from build123d import *

# Parameters (mm, degrees)
SKETCH1_W               = 154.5
SKETCH1_H               = 30
SKETCH1_W_2             = 34.5
SKETCH1_H_2             = 20
BOSS_EXTRUDE2_DEPTH     = 1
BOSS_EXTRUDE5_DEPTH     = 24
SKETCH5_W               = 3.2
SKETCH5_H               = 10
SKETCH5_H_2             = 8
SKETCH5_H_3             = 6
SKETCH5_H_4             = 4
SKETCH5_W_2             = 3
BOSS_EXTRUDE6_DEPTH     = 24
SKETCH6_W               = 28.5
SKETCH6_H               = 20
BOSS_EXTRUDE7_DEPTH     = 15
BOSS_EXTRUDE8_DEPTH     = 10
SKETCH9_W               = 8
SKETCH9_H               = 3
BOSS_EXTRUDE9_DEPTH     = 25
SKETCH10_R              = 2
CUT_EXTRUDE1_DEPTH      = 8
SKETCH11_W              = 32
SKETCH11_H              = 24
SKETCH11_W_2            = 34.7
CUT_EXTRUDE2_DEPTH      = 8
FILLET1_R               = 10
SKETCH13_W              = 15
SKETCH13_H              = 6
BOSS_EXTRUDE10_DEPTH    = 25
SKETCH15_W              = 6.4
SKETCH15_H              = 5
CUT_EXTRUDE3_DEPTH      = 7
CUT_EXTRUDE4_DEPTH      = 170.470498908
CUT_EXTRUDE4_DEPTH_BACK = 170.470498908
CHAMFER1_SIZE           = 6
SKETCH17_W              = 34.5
SKETCH17_H              = 3
BOSS_EXTRUDE11_DEPTH    = 10
CHAMFER2_SIZE           = 10


# Some blends are built 0.0001 mm under size
with BuildPart() as part:
    # Sketch1 → Boss-Extrude2 (new body)
    with BuildSketch(Plane(origin=(0, 0, 0), x_dir=(1, 0, 0), z_dir=(0, 1, 0))):
        with Locations((77.25, 15)):
            Rectangle(SKETCH1_W, SKETCH1_H)
        with Locations((137.25, -10)):
            Rectangle(SKETCH1_W_2, SKETCH1_H_2)
    extrude(amount=BOSS_EXTRUDE2_DEPTH)

    # Sketch2 → Boss-Extrude5 (add)
    with BuildSketch(Plane(origin=(0, 1, 0), x_dir=(1, 0, 0), z_dir=(0, 1, 0))):
        Polygon((3, 27), (0, 27), (0, 30), (154.5, 30), (154.5, 27), (151.5, 27), align=None)
        Polygon((0, 0), (120, 0), (120, -20), (154.5, -20), (154.5, 3), (151.5, 3), (151.5, -17), (123, -17), (123, 3), (3, 3), (0, 3), align=None)
    extrude(amount=BOSS_EXTRUDE5_DEPTH)

    # Sketch5 → Boss-Extrude6 (add)
    with BuildSketch(Plane.XY.offset(-27)):
        with Locations((9.6, 6)):
            Rectangle(SKETCH5_W, SKETCH5_H)
        with Locations((44.8, 5)):
            Rectangle(SKETCH5_W, SKETCH5_H_2)
        with Locations((80, 4)):
            Rectangle(SKETCH5_W, SKETCH5_H_3)
        with Locations((115.2, 3)):
            Rectangle(SKETCH5_W, SKETCH5_H_4)
        with Locations((153, 3)):
            Rectangle(SKETCH5_W_2, SKETCH5_H_4)
    extrude(amount=BOSS_EXTRUDE6_DEPTH)

    # Sketch6 → Boss-Extrude7 (add)
    with BuildSketch(Plane(origin=(0, 1, 0), x_dir=(1, 0, 0), z_dir=(0, 1, 0))):
        with Locations((137.25, -7)):
            Rectangle(SKETCH6_W, SKETCH6_H)
    extrude(amount=BOSS_EXTRUDE7_DEPTH)

    # Sketch7 → Boss-Extrude8 (add)
    with BuildSketch(Plane(origin=(0, 25, 0), x_dir=(1, 0, 0), z_dir=(0, 1, 0))):
        Polygon((110, 3), (110, 0), (122, 0), (122, -20), (152.5, -20), (152.5, 0), (162.5, 0), (162.5, 3), (151.5, 3), (151.5, -17), (123, -17), (123, 3), align=None)
    extrude(amount=BOSS_EXTRUDE8_DEPTH)

    # Sketch9 → Boss-Extrude9 (add)
    with BuildSketch(Plane.XZ.offset(-25)):
        with Locations((158.5, -1.5)):
            Rectangle(SKETCH9_W, SKETCH9_H)
    extrude(amount=BOSS_EXTRUDE9_DEPTH)

    # Sketch10 → Cut-Extrude1 (cut)
    with BuildSketch(Plane(origin=(0, 0, -3), x_dir=(-1, 0, 0), z_dir=(0, 0, -1))):
        with Locations((-120, 30)):
            Circle(SKETCH10_R)
        with Locations((-154.5, 30)):
            Circle(SKETCH10_R)
    extrude(amount=-CUT_EXTRUDE1_DEPTH, mode=Mode.SUBTRACT)

    # Sketch11 → Cut-Extrude2 (cut)
    with BuildSketch(Plane(origin=(0, 1, 0), x_dir=(1, 0, 0), z_dir=(0, 1, 0))):
        with Locations((27.2, 15)):
            Rectangle(SKETCH11_W, SKETCH11_H)
        with Locations((62.4, 15)):
            Rectangle(SKETCH11_W, SKETCH11_H)
        with Locations((97.6, 15)):
            Rectangle(SKETCH11_W, SKETCH11_H)
        with Locations((134.15, 15)):
            Rectangle(SKETCH11_W_2, SKETCH11_H)
    extrude(amount=-CUT_EXTRUDE2_DEPTH, mode=Mode.SUBTRACT)

    # Fillet1
    # the kernel refuses this fillet: 10 mm, written as the material it adds along each edge
    with BuildSketch(Plane(origin=(46.4, 0, -3), x_dir=(1, 0, 0), z_dir=(0, 1, 0)), Plane(origin=(43.2, 9, -3), x_dir=(-1, 0, 0), z_dir=(0, -1, 0)), Plane(origin=(46.4, 9, -27), x_dir=(1, 0, 0), z_dir=(0, -1, 0))) as fillet1_piece_1:
        with BuildLine():
            CenterArc((FILLET1_R, FILLET1_R), FILLET1_R, 180, 90)
            Line((0, FILLET1_R), (0, 0))
            Line((0, 0), (FILLET1_R, 0))
        make_face()
    extrude(amount=9)
    with BuildSketch(Plane(origin=(81.6, 0, -3), x_dir=(1, 0, 0), z_dir=(0, 1, 0)), Plane(origin=(78.4, 0, -27), x_dir=(-1, 0, 0), z_dir=(0, 1, 0)), Plane(origin=(78.4, 7, -3), x_dir=(-1, 0, 0), z_dir=(0, -1, 0)), Plane(origin=(81.6, 7, -27), x_dir=(1, 0, 0), z_dir=(0, -1, 0))) as fillet1_piece_2:
        with BuildLine():
            CenterArc((FILLET1_R, FILLET1_R), FILLET1_R, 180, 90)
            Line((0, FILLET1_R), (0, 0))
            Line((0, 0), (FILLET1_R, 0))
        make_face()
    extrude(amount=7)
    with BuildSketch(Plane(origin=(116.8, 0, -3), x_dir=(1, 0, 0), z_dir=(0, 1, 0)), Plane(origin=(113.6, 0, -27), x_dir=(-1, 0, 0), z_dir=(0, 1, 0)), Plane(origin=(113.6, 5, -3), x_dir=(-1, 0, 0), z_dir=(0, -1, 0))) as fillet1_piece_3:
        with BuildLine():
            CenterArc((FILLET1_R, FILLET1_R), FILLET1_R, 180, 90)
            Line((0, FILLET1_R), (0, 0))
            Line((0, 0), (FILLET1_R, 0))
        make_face()
    extrude(amount=5)
    with BuildSketch(Plane(origin=(43.2, 9, -27), x_dir=(-1, 0, 0), z_dir=(0, -1, 0))) as fillet1_piece_4:
        with BuildLine():
            CenterArc((FILLET1_R, -FILLET1_R), FILLET1_R, 90, 90)
            Line((0, -FILLET1_R), (0, 0))
            Line((0, 0), (FILLET1_R, 0))
        make_face()
    extrude(amount=9)
    with BuildSketch(Plane(origin=(116.8, 5, -27), x_dir=(0, 0, 1), z_dir=(0, -1, 0))) as fillet1_piece_5:
        with BuildLine():
            CenterArc((FILLET1_R, -FILLET1_R), FILLET1_R, 90, 90)
            Line((0, -FILLET1_R), (0, 0))
            Line((0, 0), (FILLET1_R, 0))
        make_face()
    extrude(amount=5)
    # the kernel refuses this fillet: 10 mm, written as the material it takes off along each edge
    with BuildSketch(Plane(origin=(154.5, 25, 35), x_dir=(0, -1, 0), z_dir=(0, 0, -1))) as fillet1_2_piece_1:
        with BuildLine():
            CenterArc((6, 10), FILLET1_R, 233.130102354, 36.869897646)
            Line((0, 2), (0, 0))
            Line((0, 0), (6, 0))
        make_face()
    extrude(amount=35, mode=Mode.SUBTRACT)
    with BuildSketch(Plane(origin=(120, 25, 0), x_dir=(1, 0, 0), z_dir=(0, 0, 1))) as fillet1_2_piece_2:
        with BuildLine():
            CenterArc((10, -6), FILLET1_R, 143.130102354, 36.869897646)
            Line((0, -6), (0, 0))
            Line((0, 0), (2, 0))
        make_face()
    extrude(amount=35, mode=Mode.SUBTRACT)

    # Sketch13 → Boss-Extrude10 (add)
    with BuildSketch(Plane.XZ):
        with Locations((7.5, 3)):
            Rectangle(SKETCH13_W, SKETCH13_H)
    boss_extrude10 = extrude(amount=-BOSS_EXTRUDE10_DEPTH)

    # Sketch15 → Cut-Extrude3 (cut)
    with BuildSketch(Plane(origin=(0, 25, 0), x_dir=(1, 0, 0), z_dir=(0, 1, 0))):
        with Locations((7.5, 0.5)):
            Rectangle(SKETCH15_W, SKETCH15_H)
    cut_extrude3 = extrude(amount=-CUT_EXTRUDE3_DEPTH, mode=Mode.SUBTRACT)

    # Mirror1: Boss-Extrude10, Cut-Extrude3 across plane
    add(boss_extrude10.mirror(Plane.XY.offset(-15)))
    add(cut_extrude3.mirror(Plane.XY.offset(-15)), mode=Mode.SUBTRACT)

    # Sketch16 → Cut-Extrude4 (cut, two sides: drawn at the far end of the back side and taken through both)
    with BuildSketch(Plane(origin=(0, 0, -3), x_dir=(-1, 0, 0), z_dir=(0, 0, -1)).offset(-CUT_EXTRUDE4_DEPTH_BACK)):
        Polygon((-8, 11), (0, 18), (0, 0), (-8, 0), align=None)
    extrude(amount=CUT_EXTRUDE4_DEPTH + CUT_EXTRUDE4_DEPTH_BACK, mode=Mode.SUBTRACT)

    # Chamfer1
    chamfer1_edges = [part.edges().sort_by_distance(p)[0] for p in [
        (15, 12.5, -30),
        (15, 12.5, 0),
    ]]
    chamfer(chamfer1_edges, length=CHAMFER1_SIZE - 0.0001)  # a hair under: the kernel refuses the full size

    # Sketch17 → Boss-Extrude11 (add)
    with BuildSketch(Plane(origin=(0, 25, 0), x_dir=(1, 0, 0), z_dir=(0, 1, 0))):
        with Locations((137.25, 28.5)):
            Rectangle(SKETCH17_W, SKETCH17_H)
    extrude(amount=BOSS_EXTRUDE11_DEPTH)

    # Chamfer2
    chamfer2_edges = [part.edges().sort_by_distance(p)[0] for p in [
        (120, 25, -28.5),
    ]]
    chamfer(chamfer2_edges, length=CHAMFER2_SIZE - 0.0001)  # a hair under: the kernel refuses the full size


solid = part.part
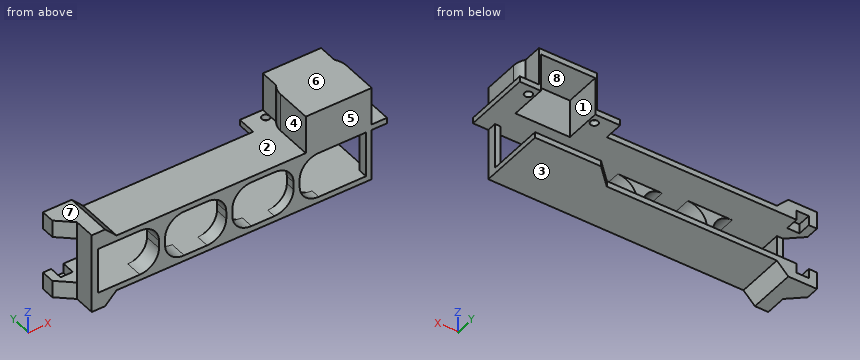
Input: part model. Units: mm. Frame: model coordinates. Face numbers are marked on the shaded views. A direction names the side the tool comes from. Give positions to 0.01 mm unless a question says otherwise; leave off trailing zeros. Write each loop counter-clockwise with the first axis right and the second up, starting at its lowest first coordinate (ties: lowest second). Pieces come first, ordered by that corner, then holes. Notation, with made-up numbers: M -22.75,70.5 L 8.25,70.5 A16 cw 8.25,90.5 Z; hole C 14.5,-10.5 d2. An arc over 180 degrees is marked long. Use one line per item in the form item = value.
1. Reachability of the marked faces 4, 5, 6, 7 and 8 from +Z, -Z, +X, -X, +Y, -Y: full face, straight path, thin tool, end or side. Return the list, or none.
Outcome:
face_4 = +Z, +Y, -Y
face_5 = +Z, -Z, +X, -X, -Y
face_6 = +Z, +X, -X, +Y, -Y
face_7 = +Z, -X, +Y, -Y
face_8 = +Y
2. Ray query, L1, parallel to Z at x = 90, y = 19; L2, parallel to Z at x = 15, y = 21.5; L3, parallel to Y at x = 154.5, z = -1.5. Return the intervals inside material, ascending.
Outcome:
L1 = -30 to -27, -3 to 0
L2 = -36 to -27, -3 to 6
L3 = 0 to 28, 32 to 35
3. Cut plane D-D on x = 75.5. Return loops of the section in (y, z), and give its area (3 significant figures).
Outcome:
outline = M 0,-30 L 25,-30 L 25,-27 L 7,-27 L 7,-24.04 L 0,-24.04 Z; M 0,-5.96 L 7,-5.96 L 7,-3 L 25,-3 L 25,0 L 0,0 Z
area = 191 mm²
4. First-contact query: P1, Ø3, axis at x = 52, y = 24, coming from the +Z side; P2, Ø18.5, axis at x = 80.5, z = -18.5, coming from the +Y side; P3, Ø5.5, axis at x = 7.5, z = -1, coming from the +Y side. Flat tips, straight axial feed; report the tip coordinate or a pass-through.
Outcome:
P1 = 0
P2 = 25
P3 = 18
5. Mould query, pull axis Z, two halves, no side actions, for the marked faces 1, 2 and 3. Classes: released by +Z, released by -Z, zero draft, split by the parting line, or undercut.
Outcome:
face_1 = undercut
face_2 = released by +Z
face_3 = released by -Z
6. Cut plane A-A on x = 132.5. Return loops of the section in (y, z), and give its area (3 significant figures).
Outcome:
outline = M 0,-30 L 35,-30 L 35,-27 L 0,-27 Z; M 0,-3 L 16,-3 L 16,17 L 35,17 L 35,20 L 0,20 Z
area = 530 mm²
7. Cut plane C-C on z = 13.5. Return loops of the section in (x, y).
Outcome:
outline = M 120,0 L 154.5,0 L 154.5,19 A10 ccw 152.5,25 L 152.5,35 L 151.5,35 L 151.5,16 L 123,16 L 123,35 L 122,35 L 122,25 A10 ccw 120,19 Z
8. Cut plane B-B on z = -10. Return loops of the section in (x, y).
Outcome:
outline = M 8,0 L 11.2,0 L 11.2,11 L 8,11 Z; M 42.74,0 L 46.86,0 L 46.86,9 L 42.74,9 Z; M 77.94,0 L 82.06,0 L 82.06,7 L 77.94,7 Z; M 113.14,0 L 117.26,0 L 117.26,5 L 113.14,5 Z; M 151.5,0 L 154.5,0 L 154.5,5 L 151.5,5 Z
